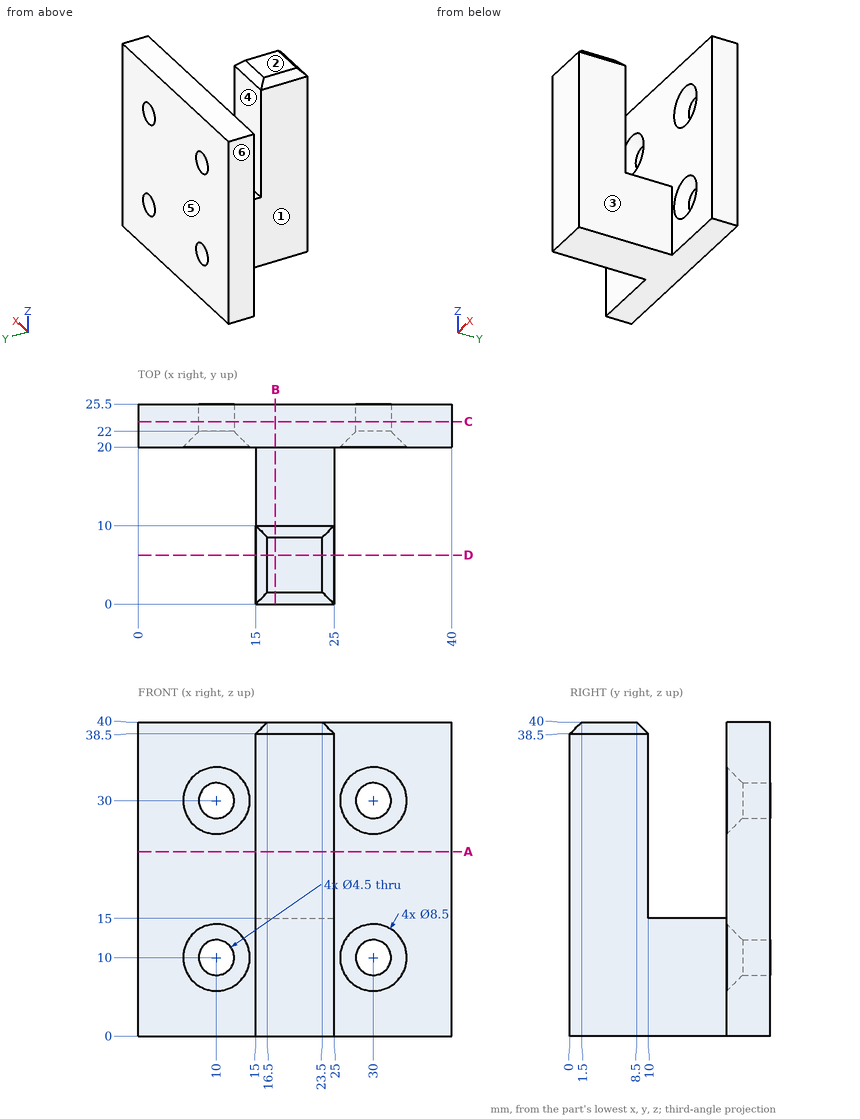
Geometry check sheet. Reference: drawing and pictorial views, mm from the part's lowest x, y, z. A direction names the side the tool comes from. Round coordinates to 2 decimals unless told otherwise and drop trailing zeros. Loops run counter-clockwise (first coordinate to the right, second up) from the corner with the lowest first, then second, coordinate; pieces in that order, holes last. Notation, with made-up numbers: (53, -32.75) -> (60, -32.75) arc R17 cw to (60, -20.75) -> close; hole circle Ø5 at (86, 34). An arc over 180 degrees is marked (long way). Answer as a JSON object with one key per item and string values. Group by question number.
Item 1: Set-up check for the marked faces 1, 2 and 3: record each of +Z, -Z, +X, -X, +Y, -Y from which the full face is reachable in a straight line by a thin tool's end or side.
Item 2: Release check for a two-part mould opening along Y. For the marked faces 4, 5 and 6 record: pulls with the +Y half, pulls with the -Y half, needs draft (parallel to the pull), parting line crosses it, or undercut.
Item 3: Cross-section at A-A, the plane z = 23.5. Record the cut outline in (x, y).
Item 4: Cross-section at D-D, the plane y = 6.25. Record the cut outline in (x, z), plus the area to 3 significant figures.
Item 5: Cross-section at B-B, the plane x = 17.5. Record the cut outline in (y, z), plus the area to 3 significant figures.
Item 6: Thickness scan on line 1 along Y through (x, z) = (17.5, 38); line 2 along Y through (x, z) = (32, 14); line 3 along X through (y, z) = (6.75, 7). Record the ranges inside material, lowest first.
Item 7: Depth check by flat-ended pin: pin 1 Ø10 at (y, z) = (8, 25.5) entering from +X; pin 2 Ø4 at (y, z) = (13.5, 22.5) entering from -X; pin 3 Ø1.5 at (x, z) = (12.5, 23.5) entering from -Y; pin 4 Ø6 at (y, z) = (10.5, 29) entering from -X. Enter the tip coordinate at first touch or a pass-through.
Item 8: Cross-section at C-C, the plane y = 23.25. Record the cut outline in (x, z).
Determined:
{
 "1": {"face 1": "+Z, -Z, -X, -Y", "face 2": "+Z, +X, -X, +Y, -Y", "face 3": "+Z, -Z, +X, -Y"},
 "2": {"face 4": "undercut", "face 5": "pulls with the +Y half", "face 6": "needs draft"},
 "3": {"outline": "(0, 20) -> (40, 20) -> (40, 25.5) -> (0, 25.5) -> close; (15, 0) -> (25, 0) -> (25, 10) -> (15, 10) -> close"},
 "4": {"outline": "(15, 0) -> (25, 0) -> (25, 38.5) -> (23.5, 40) -> (16.5, 40) -> (15, 38.5) -> close", "area": "398 mm²"},
 "5": {"outline": "(0, 0) -> (25.5, 0) -> (25.5, 40) -> (20, 40) -> (20, 15) -> (10, 15) -> (10, 38.5) -> (8.5, 40) -> (1.5, 40) -> (0, 38.5) -> close", "area": "768 mm²"},
 "6": {"line 1": "y = 0 to 10, 20 to 25.5", "line 2": "y = 20 to 25.5", "line 3": "x = 15 to 25"},
 "7": {"pin 1": "stops at x = 25", "pin 2": "passes through", "pin 3": "stops at y = 20", "pin 4": "stops at x = 15"},
 "8": {"outline": "(0, 0) -> (40, 0) -> (40, 40) -> (0, 40) -> close; hole circle Ø4.5 at (10, 10); hole circle Ø4.5 at (10, 30); hole circle Ø4.5 at (30, 10); hole circle Ø4.5 at (30, 30)"}
}
